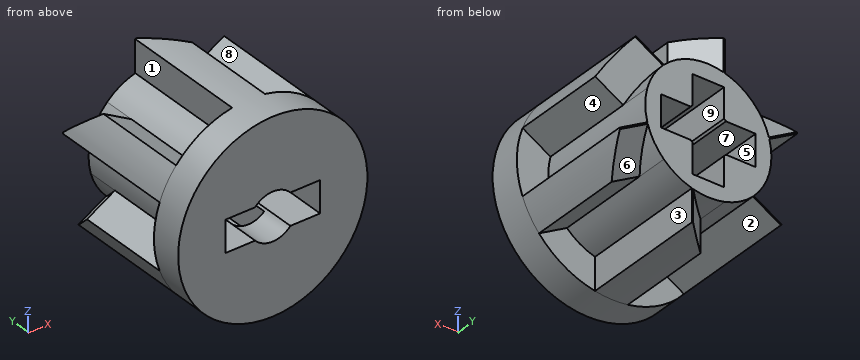
from build123d import *

# Parameters (mm, degrees)
SKETCH1_R           = 6
BOSS_EXTRUDE1_DEPTH = 2
SKETCH2_R           = 4
BOSS_EXTRUDE2_DEPTH = 8
SKETCH3_W           = 6
SKETCH3_H           = 2
CUT_EXTRUDE1_DEPTH  = 14.114877049
SKETCH4_W           = 2
SKETCH4_H           = 6
CUT_EXTRUDE2_DEPTH  = 8
SKETCH10_R          = 1.5
CUT_EXTRUDE3_DEPTH  = 14.114877049
BOSS_EXTRUDE3_START = -8
BOSS_EXTRUDE3_DEPTH = 8
CHAMFER3_SIZE       = 2


with BuildPart() as part:
    # Sketch1 → Boss-Extrude1 (new body)
    with BuildSketch(Plane(origin=(0, 0, 0), x_dir=(1, 0, 0), z_dir=(0, 1, 0))):
        with Locations(Location((0, 0, 0), (0, 0, 270))):
            Circle(SKETCH1_R)
    extrude(amount=BOSS_EXTRUDE1_DEPTH)

    # Sketch2 → Boss-Extrude2 (add)
    with BuildSketch(Plane(origin=(0, 2, 0), x_dir=(1, 0, 0), z_dir=(0, 1, 0))):
        with Locations(Location((0, 0, 0), (0, 0, 270))):
            Circle(SKETCH2_R)
    extrude(amount=BOSS_EXTRUDE2_DEPTH)

    # Sketch3 → Cut-Extrude1 (cut, through all)
    with BuildSketch(Plane(origin=(0, 10, 0), x_dir=(1, 0, 0), z_dir=(0, 1, 0))):
        Rectangle(SKETCH3_W, SKETCH3_H)
    extrude(amount=-CUT_EXTRUDE1_DEPTH, mode=Mode.SUBTRACT)

    # Sketch4 → Cut-Extrude2 (cut)
    with BuildSketch(Plane(origin=(0, 10, 0), x_dir=(1, 0, 0), z_dir=(0, 1, 0))):
        Rectangle(SKETCH4_W, SKETCH4_H)
    extrude(amount=-CUT_EXTRUDE2_DEPTH, mode=Mode.SUBTRACT)

    # Sketch10 → Cut-Extrude3 (cut, through all)
    with BuildSketch(Plane(origin=(0, 10, 0), x_dir=(1, 0, 0), z_dir=(0, 1, 0))):
        Circle(SKETCH10_R)
    extrude(amount=-CUT_EXTRUDE3_DEPTH, mode=Mode.SUBTRACT)

    # Sketch11 → Boss-Extrude3 (add)
    with BuildSketch(Plane(origin=(0, 10, 0), x_dir=(1, 0, 0), z_dir=(0, 1, 0)).offset(BOSS_EXTRUDE3_START)):
        with BuildLine():
            Line((-1.041889066, 5.908846518), (-1.042680136, 3.861711814))
            Line((-1.042680136, 3.861711814), (1.041889066, 3.86192532))
            Line((1.041889066, 3.86192532), (1.041889066, 5.908846518))
            ThreePointArc((1.041889066, 5.908846518), (0, 6), (-1.041889066, 5.908846518))
        make_face()
        with BuildLine():
            Line((4.596266659, 3.856725658), (2.823000465, 2.833843393))
            Line((2.823000465, 2.833843393), (3.865469967, 1.028660261))
            Line((3.865469967, 1.028660261), (5.638155725, 2.05212086))
            ThreePointArc((5.638155725, 2.05212086), (5.196152423, 3), (4.596266659, 3.856725658))
        make_face()
        with BuildLine():
            Line((5.638155725, -2.05212086), (3.865680601, -1.027868421))
            Line((3.865680601, -1.027868421), (2.823580901, -2.833265059))
            Line((2.823580901, -2.833265059), (4.596266659, -3.856725658))
            ThreePointArc((4.596266659, -3.856725658), (5.196152423, -3), (5.638155725, -2.05212086))
        make_face()
        with BuildLine():
            Line((1.041889066, -5.908846518), (1.042680136, -3.861711814))
            Line((1.042680136, -3.861711814), (-1.041889066, -3.86192532))
            Line((-1.041889066, -3.86192532), (-1.041889066, -5.908846518))
            ThreePointArc((-1.041889066, -5.908846518), (0, -6), (1.041889066, -5.908846518))
        make_face()
        with BuildLine():
            Line((-4.596266659, -3.856725658), (-2.823000465, -2.833843393))
            Line((-2.823000465, -2.833843393), (-3.865469967, -1.028660261))
            Line((-3.865469967, -1.028660261), (-5.638155725, -2.05212086))
            ThreePointArc((-5.638155725, -2.05212086), (-5.196152423, -3), (-4.596266659, -3.856725658))
        make_face()
        with BuildLine():
            Line((-5.638155725, 2.05212086), (-3.865680601, 1.027868421))
            Line((-3.865680601, 1.027868421), (-2.823580901, 2.833265059))
            Line((-2.823580901, 2.833265059), (-4.596266659, 3.856725658))
            ThreePointArc((-4.596266659, 3.856725658), (-5.196152423, 3), (-5.638155725, 2.05212086))
        make_face()
    extrude(amount=BOSS_EXTRUDE3_DEPTH)

    # Chamfer3
    # the kernel refuses this chamfer: 2 mm, written as the material it takes off along each edge
    with BuildSketch(Plane(origin=(9.051545693, 10, -6.426687193), x_dir=(0.49947639120581244, 0.02749587661058648, 0.865891050535478), z_dir=(-0.8662185531215343, 0, 0.49966530620810146))) as chamfer3_piece_1_section:
        Polygon((CHAMFER3_SIZE * 0.999621916911, -CHAMFER3_SIZE * 0.0274958766106), (-CHAMFER3_SIZE * 0.0274958766106, -CHAMFER3_SIZE * 0.999621916911), (0, 0), align=None)
    chamfer3_piece_1 = extrude(amount=12.333866809, mode=Mode.PRIVATE)
    chamfer3_piece_1 = chamfer3_piece_1 - Plane(origin=(0, 9.335728608, 0), x_dir=(0, 0, 1), z_dir=(0, -1, 0)) * Cylinder(4, 33, mode=Mode.PRIVATE)
    add(chamfer3_piece_1, mode=Mode.SUBTRACT)
    with BuildSketch(Plane(origin=(10.091447218, 10, 4.625524917), x_dir=(-0.5001454510704151, 0.027495876610586487, 0.8655047686425457), z_dir=(-0.8658321251267121, 0, -0.5003346191286003))) as chamfer3_piece_2_section:
        Polygon((CHAMFER3_SIZE * 0.999621916911, -CHAMFER3_SIZE * 0.0274958766106), (-CHAMFER3_SIZE * 0.0274958766106, -CHAMFER3_SIZE * 0.999621916911), (0, 0), align=None)
    chamfer3_piece_2 = extrude(amount=12.333866809, mode=Mode.PRIVATE)
    chamfer3_piece_2 = chamfer3_piece_2 - Plane(origin=(0, 9.332082239, 0), x_dir=(0, 0, 1), z_dir=(0, -1, 0)) * Cylinder(4, 33, mode=Mode.PRIVATE)
    add(chamfer3_piece_2, mode=Mode.SUBTRACT)
    with BuildSketch(Plane(origin=(1.039901525, 10, 11.05221211), x_dir=(0.027495874557653455, -0.9996219169112968, 1.0625176464596534e-05), z_dir=(0.0003864279948254377, 0, -0.9999999253366997))) as chamfer3_piece_3_section:
        Polygon((CHAMFER3_SIZE * 0.999621916911, CHAMFER3_SIZE * 0.0274958766106), (-CHAMFER3_SIZE * 0.0274958766106, CHAMFER3_SIZE * 0.999621916911), (0, 0), align=None)
    chamfer3_piece_3 = extrude(amount=12.333866809, mode=Mode.PRIVATE)
    chamfer3_piece_3 = chamfer3_piece_3 - Plane(origin=(0, 9.010529582, 0), x_dir=(0, 0, 1), z_dir=(0, -1, 0)) * Cylinder(4, 33, mode=Mode.PRIVATE)
    add(chamfer3_piece_3, mode=Mode.SUBTRACT)
    with BuildSketch(Plane(origin=(-9.051545693, 10, 6.426687193), x_dir=(-0.4994763912058064, 0.02749587661058648, -0.8658910505354813), z_dir=(0.8662185531215377, 0, -0.4996653062080955))) as chamfer3_piece_4_section:
        Polygon((CHAMFER3_SIZE * 0.999621916911, -CHAMFER3_SIZE * 0.0274958766106), (-CHAMFER3_SIZE * 0.0274958766106, -CHAMFER3_SIZE * 0.999621916911), (0, 0), align=None)
    chamfer3_piece_4 = extrude(amount=12.333866809, mode=Mode.PRIVATE)
    chamfer3_piece_4 = chamfer3_piece_4 - Plane(origin=(0, 9.335728608, 0), x_dir=(0, 0, 1), z_dir=(0, -1, 0)) * Cylinder(4, 33, mode=Mode.PRIVATE)
    add(chamfer3_piece_4, mode=Mode.SUBTRACT)
    with BuildSketch(Plane(origin=(-10.091447218, 10, -4.625524917), x_dir=(0.5001454510704163, 0.02749587661058648, -0.8655047686425448), z_dir=(0.8658321251267114, 0, 0.5003346191286018))) as chamfer3_piece_5_section:
        Polygon((CHAMFER3_SIZE * 0.999621916911, -CHAMFER3_SIZE * 0.0274958766106), (-CHAMFER3_SIZE * 0.0274958766106, -CHAMFER3_SIZE * 0.999621916911), (0, 0), align=None)
    chamfer3_piece_5 = extrude(amount=12.333866809, mode=Mode.PRIVATE)
    chamfer3_piece_5 = chamfer3_piece_5 - Plane(origin=(0, 9.332082239, 0), x_dir=(0, 0, 1), z_dir=(0, -1, 0)) * Cylinder(4, 33, mode=Mode.PRIVATE)
    add(chamfer3_piece_5, mode=Mode.SUBTRACT)
    with BuildSketch(Plane(origin=(-1.039901525, 10, -11.05221211), x_dir=(0.9996218422762253, 0.027495876610586487, 0.00038628189292865347), z_dir=(-0.00038642799481849587, 0, 0.9999999253366997))) as chamfer3_piece_6_section:
        Polygon((CHAMFER3_SIZE * 0.999621916911, -CHAMFER3_SIZE * 0.0274958766106), (-CHAMFER3_SIZE * 0.0274958766106, -CHAMFER3_SIZE * 0.999621916911), (0, 0), align=None)
    chamfer3_piece_6 = extrude(amount=12.333866809, mode=Mode.PRIVATE)
    chamfer3_piece_6 = chamfer3_piece_6 - Plane(origin=(0, 9.346435038, 0), x_dir=(0, 0, 1), z_dir=(0, -1, 0)) * Cylinder(4, 33, mode=Mode.PRIVATE)
    add(chamfer3_piece_6, mode=Mode.SUBTRACT)


solid = part.part
The listing builds one solid part. Answer for the finished solid, in the listing's coordinates (mm). Face numbers are marked on the shaded views. A direction names the side the tool comes from. Give positions to 0.01 mm unless a question says otherwise; leave off trailing zeros. Write each loop counter-clockwise with the first axis right and the second up, starting at its lowest first coordinate (ties: lowest second). Pieces come first, ordered by that corner, then holes. Notation, with made-up numbers: (35, 67.25) -> (52, 67.25) arc R14 cw to (52, 73.25) -> close; hole circle Ø10 at (24.25, 16). An arc over 180 degrees is marked (long way). Use a Markdown table: item, result.
(1) Find the intervals of material crossed by probe 1 along Z at (x, y) = (0, 6.25); probe 2 along X at (y, z) = (3.75, -5.5); probe 3 along X at (y, z) = (7, 1.5), in increasing order. Write a range as from..to.
Return value:
| item | result |
|---|---|
| probe 1 | -6..-3, 3..6 |
| probe 2 | -1.04..1.04 |
| probe 3 | -4.68..-1, 1..4.68 |
(2) Section D-D, the plane x = 5 is taken. Determine the outline of the cut face in (y, z).
Return value:
| item | result |
|---|---|
| outline | (0, -3.32) -> (8.67, -3.32) -> (10, -1.78) -> (10, -1.68) -> (2, -1.68) -> (2, 1.68) -> (8, 1.68) -> (9.41, 3.32) -> (0, 3.32) -> close |
(3) For the marked faces 1, 2, 3, 4 and 5, determine the directions among +Z, -Z, +X, -X, +Y, -Y from which every point of the face is accessible in a straight line to the end or side of a thin tool.
Return value:
| item | result |
|---|---|
| face 1 | +Z, -X, +Y |
| face 2 | -Z, +Y |
| face 3 | -Z, +X, +Y |
| face 4 | +X, +Y |
| face 5 | +Y, -Y |
(4) Flat-ended cylindrical pins translate along their axes: P1, Ø1.5, axis at x = 1, y = 4.5, coming from the +Z side; P2, Ø1.5, axis at x = -2, y = 4, coming from the -Z side; P3, Ø0.6, axis at x = 0, z = -2, coming from the +Y side. Find the tip coordinate at first contact, or state that the pin passes through.
Return value:
| item | result |
|---|---|
| P1 | z = 5.99 |
| P2 | z = -3.8 |
| P3 | y = 2 |
(5) Section C-C, the plane z = 5.25 is taken. Determine the outline of the cut face in (x, y).
Return value:
| item | result |
|---|---|
| outline | (-2.9, 0) -> (2.9, 0) -> (2.9, 2) -> (1.04, 2) -> (1.04, 8) -> (-0.96, 10) -> (-1.04, 10) -> (-1.04, 2) -> (-2.9, 2) -> close |
(6) Determine the mould class of the marked faces 6, 7, 8 and 9 for opening direction Z: released by +Z, released by -Z, zero draft, split by the parting line, or undercut.
Return value:
| item | result |
|---|---|
| face 6 | released by -Z |
| face 7 | undercut |
| face 8 | released by +Z |
| face 9 | undercut |
(7) Section A-A, the plane x = 2 is taken. Determine the outline of the cut face in (y, z).
Return value:
| item | result |
|---|---|
| outline | (0, -5.66) -> (2, -5.66) -> (2, -3.46) -> (10, -3.46) -> (10, -1) -> (0, -1) -> close; (0, 1) -> (10, 1) -> (10, 3.46) -> (2, 3.46) -> (2, 5.66) -> (0, 5.66) -> close |
(8) Section B-B, the plane z = 0 is taken. Determine the outline of the cut face in (x, y), then the cut area to 3 significant figures.
Return value:
| item | result |
|---|---|
| outline | (-6, 0) -> (-3, 0) -> (-3, 10) -> (-4, 10) -> (-4, 2) -> (-6, 2) -> close; (3, 0) -> (6, 0) -> (6, 2) -> (4, 2) -> (4, 10) -> (3, 10) -> close |
| area | 28.0 mm2 |
